from build123d import *

# Parameters (mm, degrees)
BOSS_EXTRUDE1_DEPTH           = 45
SKETCH3_W                     = 30
SKETCH3_H                     = 40
CUT_EXTRUDE1_DEPTH            = 88.304481557
SKETCH4_W                     = 32
SKETCH4_H                     = 32
SKETCH4_W_2                   = 20.5
SKETCH4_H_2                   = 20.5
BOSS_EXTRUDE2_DEPTH           = 35
SKETCH6_W                     = 5
SKETCH6_H                     = 5
CUT_EXTRUDE4_DEPTH            = 35
RIB1_REACH                    = 87.394
SKETCH9_WALL_W                = 225.450736488
SKETCH9_WALL_H                = 2
LPATTERN1_COUNT               = 2
LPATTERN1_PITCH               = 20
RIB6_REACH                    = 100.659
SKETCH14_WALL_W               = 234.916193708
SKETCH14_WALL_H               = 2
RIB7_START                    = -2
RIB7_DEPTH                    = 2
FILLET2_R                     = 5
FILLET3_R                     = 5
RIB10_REACH                   = 92.525
SKETCH17_WALL_W               = 226.513312862
SKETCH17_WALL_H               = 2
RIB11_REACH                   = 92.525
SKETCH18_WALL_W               = 226.513312862
SKETCH18_WALL_H               = 2
FILLET4_R                     = 10
LPATTERN2_COUNT               = 2
LPATTERN2_PITCH               = 43
FILLET4_OF_LPATTERN2_R        = 10
M5_CLEARANCE_HOLE2_AT_2_COUNT = 2
M5_CLEARANCE_HOLE2_AT_2_PITCH = 15
M2_5_CLEARANCE_HOLE1_D        = 2.9
FILLET5_R                     = 2.5
SKETCH4_4_R                   = 2.5
BOSS_EXTRUDE4_DEPTH           = 8
CIRPATTERN1_COUNT             = 4
CHAMFER1_SIZE                 = 3
FILLET6_R                     = 5
FILLET7_R                     = 1.5


# Read off the part's stored shape, not the designer's step: Rib7
with BuildPart() as part:
    # Sketch2 → Boss-Extrude1 (new body)
    with BuildSketch(Plane.XY):
        Polygon((-53.5125, -22.5), (17.8375, -22.5), (17.8375, -17.5), (-9.5125, -17.5), (-9.5125, 22.5), (-14.5125, 22.5), (-14.5125, -17.5), (-48.5125, -17.5), (-48.5125, 22.5), (-53.5125, 22.5), align=None)
    extrude(amount=BOSS_EXTRUDE1_DEPTH)

    # Sketch3 → Cut-Extrude1 (cut, through all)
    with BuildSketch(Plane(origin=(-53.5125, 0, 0), x_dir=(0, 0, -1), z_dir=(1, 0, 0))):
        with Locations((-22.5, 2.5)):
            Rectangle(SKETCH3_W, SKETCH3_H)
    extrude(amount=CUT_EXTRUDE1_DEPTH, mode=Mode.SUBTRACT)

    # Sketch4 → Boss-Extrude2 (add)
    with BuildSketch(Plane.XZ.offset(22.5)):
        with Locations((1.8375, 22.5)):
            Rectangle(SKETCH4_W, SKETCH4_H)
        with Locations((1.8375, 22.5)):
            Rectangle(SKETCH4_W_2, SKETCH4_H_2, mode=Mode.SUBTRACT)
    extrude(amount=BOSS_EXTRUDE2_DEPTH)

    # Sketch6 → Cut-Extrude4 (cut)
    with BuildSketch(Plane(origin=(0, -57.5, 0), x_dir=(-1, 0, 0), z_dir=(0, -1, 0))):
        with Locations((11.6625, -36)):
            Rectangle(SKETCH6_W, SKETCH6_H)
        with Locations((-15.3375, -36)):
            Rectangle(SKETCH6_W, SKETCH6_H)
        with Locations((-15.3375, -9)):
            Rectangle(SKETCH6_W, SKETCH6_H)
        with Locations((11.6625, -9)):
            Rectangle(SKETCH6_W, SKETCH6_H)
    extrude(amount=-CUT_EXTRUDE4_DEPTH, mode=Mode.SUBTRACT)

    # Sketch9 wall → Rib1 (add, up to next)
    with BuildSketch(Plane(origin=(-33.8375, -40, 33.5), x_dir=(-0.747199752598, 0.664599525818, 0), z_dir=(-0.664599525818, -0.747199752598, 0)), mode=Mode.PRIVATE) as rib1_sk1:
        with Locations((0, 1)):
            Rectangle(SKETCH9_WALL_W, SKETCH9_WALL_H)
    rib1_tool1 = extrude(rib1_sk1.sketch, amount=-RIB1_REACH, mode=Mode.PRIVATE) - part.part
    rib1 = rib1_tool1.solids().sort_by_distance((-33.8375, -40, 33.5))[0]
    add(rib1)

    # LPattern1: Rib1 ×2
    with Locations(*[(0, 0, -i * LPATTERN1_PITCH) for i in range(1, LPATTERN1_COUNT)]):
        add(rib1)

    # Sketch14 wall → Rib6 (add, up to next)
    with BuildSketch(Plane(origin=(12.8375, -40, 3.25), x_dir=(0, 0.983188736076, -0.182592193843), z_dir=(0, 0.182592193843, 0.983188736076)), mode=Mode.PRIVATE) as rib6_sk1:
        with Locations((0, 1)):
            Rectangle(SKETCH14_WALL_W, SKETCH14_WALL_H)
    rib6_tool1 = extrude(rib6_sk1.sketch, amount=RIB6_REACH, mode=Mode.PRIVATE) - part.part
    rib6 = rib6_tool1.solids().sort_by_distance((12.8375, -40, 3.25))[0]
    add(rib6)

    # Rib7 outline → Rib7 (add)
    with BuildSketch(Plane.ZY.offset(9.1625).offset(RIB7_START)):
        Polygon((0, -22.5), (6.5, -57.5), (6.5, -22.5), align=None)
    rib7 = extrude(amount=RIB7_DEPTH)

    # Fillet2
    fillet2_edges = [part.edges().sort_by_distance(p)[0] for p in [
        (1.8375, -22.5, 38.5),
        (-14.1625, -22.5, 22.5),
        (1.8375, -22.5, 6.5),
    ]]
    fillet(fillet2_edges, radius=FILLET2_R)

    # Fillet3
    fillet3_edges = [part.edges().sort_by_distance(p)[0] for p in [
        (-9.5125, -17.5, 41.25),
        (-9.5125, -17.5, 3.75),
    ]]
    fillet(fillet3_edges, radius=FILLET3_R)

    # Sketch17 wall → Rib10 (add, up to next)
    with BuildSketch(Plane(origin=(-40.0125, 2.5, 45), x_dir=(0.391140640345, -0.920330918458, 0), z_dir=(0.920330918458, 0.391140640345, 0)), mode=Mode.PRIVATE) as rib10_sk1:
        with Locations((0, 1)):
            Rectangle(SKETCH17_WALL_W, SKETCH17_WALL_H)
    rib10_tool1 = extrude(rib10_sk1.sketch, amount=-RIB10_REACH, mode=Mode.PRIVATE) - part.part
    rib10 = rib10_tool1.solids().sort_by_distance((-40.0125, 2.5, 45))[0]
    add(rib10)

    # Sketch18 wall → Rib11 (add, up to next)
    with BuildSketch(Plane(origin=(-23.0125, 2.5, 45), x_dir=(0.391140640345, 0.920330918458, 0), z_dir=(-0.920330918458, 0.391140640345, 0)), mode=Mode.PRIVATE) as rib11_sk1:
        with Locations((0, 1)):
            Rectangle(SKETCH18_WALL_W, SKETCH18_WALL_H)
    rib11_tool1 = extrude(rib11_sk1.sketch, amount=-RIB11_REACH, mode=Mode.PRIVATE) - part.part
    rib11 = rib11_tool1.solids().sort_by_distance((-23.0125, 2.5, 45))[0]
    add(rib11)

    # Fillet4
    # the kernel refuses this fillet: 10 mm, written as the material it adds along each edge
    with BuildSketch(Plane(origin=(-31.5125, -17.5, 45), x_dir=(-0.391140640345148, 0.9203309184583486, 0), z_dir=(0, 0, -1))) as fillet4_piece_1:
        with BuildLine():
            CenterArc((FILLET4_R * 2.35294117647, FILLET4_R), FILLET4_R, 136.050984017, 133.949015983)
            Line((FILLET4_R * 1.63298352692, FILLET4_R * 1.69401799894), (0, 0))
            Line((0, 0), (FILLET4_R * 2.35294117647, 0))
        make_face()
    extrude(amount=2)

    # LPattern2: Rib10, Rib11 ×2
    with Locations(*[(0, 0, -i * LPATTERN2_PITCH) for i in range(1, LPATTERN2_COUNT)]):
        add(rib10)
        add(rib11)

    # Fillet4 of LPattern2
    # the kernel refuses this fillet: 10 mm, written as the material it adds along each edge
    with BuildSketch(Plane(origin=(-31.5125, -17.5, 60.823529412), x_dir=(-0.39114064034514817, 0.9203309184583486, 0), z_dir=(0, 0, -1))) as fillet4_of_lpattern2_piece_1_section:
        with BuildLine():
            CenterArc((FILLET4_OF_LPATTERN2_R * 2.35294117647, FILLET4_OF_LPATTERN2_R), FILLET4_OF_LPATTERN2_R, 136.050984017, 133.949015983)
            Line((FILLET4_OF_LPATTERN2_R * 1.63298352692, FILLET4_OF_LPATTERN2_R * 1.69401799894), (0, 0))
            Line((0, 0), (FILLET4_OF_LPATTERN2_R * 2.35294117647, 0))
        make_face()
    fillet4_of_lpattern2_piece_1 = extrude(amount=60.823529412, mode=Mode.PRIVATE)
    fillet4_of_lpattern2_piece_1 = split(fillet4_of_lpattern2_piece_1, bisect_by=Plane(origin=(-31.5125, -6.311496297, 43), z_dir=(0, 0, 1)), keep=Keep.TOP, mode=Mode.PRIVATE)
    fillet4_of_lpattern2_piece_1 = split(fillet4_of_lpattern2_piece_1, bisect_by=Plane(origin=(-31.5125, -6.311496297, 45), z_dir=(0, 0, -1)), keep=Keep.TOP, mode=Mode.PRIVATE)
    add(fillet4_of_lpattern2_piece_1)
    with BuildSketch(Plane(origin=(-31.5125, -17.5, 2), x_dir=(-0.391140640345148, 0.9203309184583486, 0), z_dir=(0, 0, -1))) as fillet4_of_lpattern2_piece_2:
        with BuildLine():
            CenterArc((FILLET4_OF_LPATTERN2_R * 2.35294117647, FILLET4_OF_LPATTERN2_R), FILLET4_OF_LPATTERN2_R, 136.050984017, 133.949015983)
            Line((FILLET4_OF_LPATTERN2_R * 1.63298352692, FILLET4_OF_LPATTERN2_R * 1.69401799894), (0, 0))
            Line((0, 0), (FILLET4_OF_LPATTERN2_R * 2.35294117647, 0))
        make_face()
    extrude(amount=2)

    # Sketch22 → M5 Clearance Hole2 (revolve, cut)
    with BuildSketch(Plane(origin=(1.8375, -32.5, 38.5), x_dir=(0, -1, 0), z_dir=(1, 0, 0))):
        Polygon((0, 0), (0, 7.652366702), (2.75, 6), (2.75, 0), align=None)
    m5_clearance_hole2 = revolve(axis=Axis((1.8375, -32.5, 44.85), (0, 0, -1)), mode=Mode.SUBTRACT)

    # M5 Clearance Hole2 at 2: M5 Clearance Hole2 ×2
    with Locations(*[(0, -i * M5_CLEARANCE_HOLE2_AT_2_PITCH, 0) for i in range(1, M5_CLEARANCE_HOLE2_AT_2_COUNT)]):
        add(m5_clearance_hole2, mode=Mode.SUBTRACT)

    # M2.5 Clearance Hole1 (through all)
    with Locations(Plane.ZY.offset(53.5125)):
        with Locations((5.2, 15.5), (39.8, 15.5), (39.8, -6.5), (5.2, -6.5)):
            Hole(M2_5_CLEARANCE_HOLE1_D / 2)

    # Fillet5
    fillet5_edges = [part.edges().sort_by_distance(p)[0] for p in [
        (-9.1625, -40, 11.5),
        (12.8375, -40, 11.5),
        (12.8375, -40, 33.5),
        (-9.1625, -40, 33.5),
    ]]
    fillet(fillet5_edges, radius=FILLET5_R)

    # Sketch4<4> → Boss-Extrude4 (add)
    with BuildSketch(Plane.XZ.offset(22.5)):
        with Locations(Location((1.8375, 22.5, 0), (0, 0, 180))):
            Circle(SKETCH4_4_R)
    extrude(amount=BOSS_EXTRUDE4_DEPTH)

    # CirPattern1: M5 Clearance Hole2 ×4 about axis
    cirpattern1_axis = Axis((1.8375, -30.5, 22.5), (0, -1, 0))
    for i in range(1, CIRPATTERN1_COUNT):
        add(m5_clearance_hole2.rotate(cirpattern1_axis, i * 360 / CIRPATTERN1_COUNT), mode=Mode.SUBTRACT)

    # CirPattern1 copy 1 sketch → CirPattern1 copy 1 (revolve, cut)
    with BuildSketch(Plane(origin=(-14.1625, -47.5, 22.5), x_dir=(0, -1, 0), z_dir=(0, 0, 1))):
        Polygon((0, 0), (0, 7.652366702), (2.75, 6), (2.75, 0), align=None)
    revolve(axis=Axis((-20.5125, -47.5, 22.5), (1, 0, 0)), mode=Mode.SUBTRACT)

    # CirPattern1 copy 2 sketch → CirPattern1 copy 2 (revolve, cut)
    with BuildSketch(Plane(origin=(1.8375, -47.5, 6.5), x_dir=(0, -1, 0), z_dir=(-1, 0, 0))):
        Polygon((0, 0), (0, 7.652366702), (2.75, 6), (2.75, 0), align=None)
    revolve(axis=Axis((1.8375, -47.5, 0.15), (0, 0, 1)), mode=Mode.SUBTRACT)

    # CirPattern1 copy 3 sketch → CirPattern1 copy 3 (revolve, cut)
    with BuildSketch(Plane(origin=(17.8375, -47.5, 22.5), x_dir=(0, -1, 0), z_dir=(0, 0, -1))):
        Polygon((0, 0), (0, 7.652366702), (2.75, 6), (2.75, 0), align=None)
    revolve(axis=Axis((24.1875, -47.5, 22.5), (-1, 0, 0)), mode=Mode.SUBTRACT)

    # Mirror1: Rib6, Rib7 across plane
    add(rib6.mirror(Plane.XY.offset(22.5)))
    add(rib7.mirror(Plane.XY.offset(22.5)))

    # Chamfer1
    chamfer1_edges = [part.edges().sort_by_distance(p)[0] for p in [
        (17.8375, -20, 0),
        (-12.0125, 22.5, 37.5),
        (-51.0125, 22.5, 37.5),
        (-12.0125, 22.5, 7.5),
        (-51.0125, 22.5, 7.5),
        (17.8375, -20, 45),
    ]]
    chamfer(chamfer1_edges, length=CHAMFER1_SIZE)

    # Fillet6
    fillet6_edges = [part.edges().sort_by_distance(p)[0] for p in [
        (-51.0125, -17.5, 37.5),
        (-51.0125, -17.5, 7.5),
    ]]
    fillet(fillet6_edges, radius=FILLET6_R)

    # Fillet7
    fillet7_edges = [part.edges().sort_by_distance(p)[0] for p in [
        (-9.1625, -22.5, 4.5),
        (-32.5875, -22.5, 33.5),
        (-36.3375, -22.5, 31.5),
        (-36.3375, -22.5, 13.5),
        (-14.1625, -42.5, 13.5),
        (-14.1625, -42.5, 31.5),
        (-15.626966094, -23.964466094, 13.5),
        (-15.626966094, -23.964466094, 31.5),
        (-32.5875, -22.5, 11.5),
        (-9.894733047, -22.5, 10.767766953),
        (-9.1625, -22.5, 40.5),
        (-9.894733047, -22.5, 34.232233047),
    ]]
    fillet(fillet7_edges, radius=FILLET7_R)


solid = part.part
CAD build for the part. Positions are in the model's coordinates, mm. A direction names the side the tool comes from. Give positions to 0.01 mm unless a question says otherwise; leave off trailing zeros. Loops run counter-clockwise (first coordinate to the right, second up) from the corner with the lowest first, then second, coordinate; pieces in that order, holes last. Notation, with made-up numbers: M 23.5,38.5 L 61.5,38.5 A21 ccw 61.5,60.5 Z; hole C 62,4.25 d10. An arc over 180 degrees is marked long. One line per question, with ' | ' between items. Start each with the question number.
1. Flat gauge pins, fed straight in: pin 1 (1 mm diameter, centred on x = 7, z = 26, fed in from +Y); pin 2 (6 mm diameter, centred on y = -40, z = 6.5, fed in from +X); pin 3 (3 mm diameter, centred on y = 10, z = 7, fed in from +X); pin 4 (2.5 mm diameter, centred on y = -6.5, z = 39.8, fed in from -X). Where does each tip first touch, or does it go through?
2. Saw through at C-C on y = 2. Give the cut face in (x, z).
3. Saw through at D-D on x = -37. Give the cut face in (y, z), plus the area to 3 significant figures.
4. Probe L1, parallel to X at y = -9.5, z = 41.5; L2, parallel to Z at x = -26.5, y = -13.5; L3, parallel to X at y = -33.5, z = 6. List the from-to ranges inside material, lowest first. Write a range as from..to.
5. Saw through at A-A on z = 22.5. State how many separate pieces and enclosed holes the cut face has, plus the area to 3 significant figures.
6. 3-axis set-ups, long thin cutter, end or side, ignore diameter. For faces 1 (the face through (-18, -17.5, 23)), 2 (the face through (-12, 21, 39)), 3 (the face through (15.003, -29.753, 22.621)): which of +Z, -Z, +X, -X, +Y, -Y reach the whole face in a straight line?
7. Two-plate mould, pull along Y, no slides. Class faces 4 (the face through (2, -57.5, 12)), 5 (the face through (12.838, -36, 6)), 6 (the face through (-50.98, 15.56, 41.25)): pulls with the +Y half, pulls with the -Y half, needs draft (parallel to the pull), parting line crosses it, or undercut.
Result sheet:
1) pin 1: stops at y = -17.5 | pin 2: stops at x = 12.89 | pin 3: stops at x = -9.51 | pin 4: passes through
2) outline: M -53.51,0 L -39.46,0 L -39.46,2 L -48.51,2 L -48.51,7.5 L -53.51,7.5 Z; M -53.51,37.5 L -48.51,37.5 L -48.51,43 L -39.46,43 L -39.46,45 L -53.51,45 Z; M -23.56,0 L -9.51,0 L -9.51,7.5 L -14.51,7.5 L -14.51,2 L -23.56,2 Z; M -23.56,43 L -14.51,43 L -14.51,37.5 L -9.51,37.5 L -9.51,45 L -23.56,45 Z
3) outline: M -37.19,11.5 L -24,11.5 A1.5 cw -22.5,10 L -22.5,0 L -0.29,0 L -0.29,2 L -17.5,2 L -17.5,43 L -0.29,43 L -0.29,45 L -22.5,45 L -22.5,35 A1.5 cw -24,33.5 L -37.19,33.5 L -37.19,31.5 L -24,31.5 A1.5 cw -22.5,30 L -22.5,15 A1.5 cw -24,13.5 L -37.19,13.5 Z | area: 355 mm^2
4) L1: x = -53.51..-48.51, -14.51..-9.51 | L2: z = 0..2, 43..45 | L3: x = -9.16..-7.16, 10.84..12.84
5) separate pieces: 5 | enclosed holes: 0 | area: 678 mm^2
6) face 1: +Y | face 2: +X, -X, +Y | face 3: +X
7) face 4: pulls with the -Y half | face 5: needs draft | face 6: undercut
